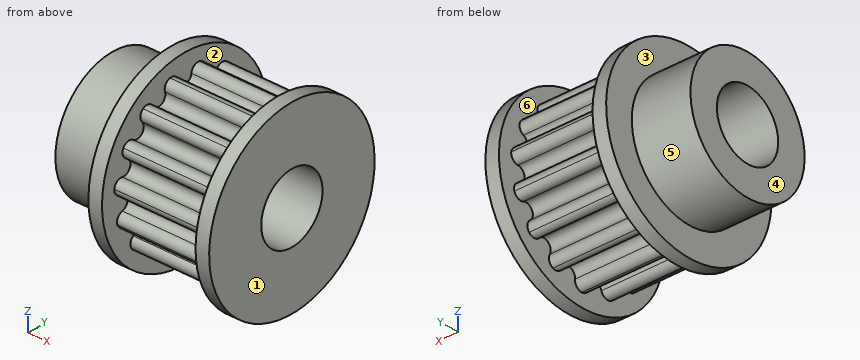
```python
from build123d import *

# Parameters (mm, degrees)
CUT_EXTRUDE1_START = 11
CUT_EXTRUDE1_DEPTH = 11


with BuildPart() as part:
    # Sketch1 → Revolve2 (revolve)
    with BuildSketch(Plane.XY, mode=Mode.PRIVATE) as revolve2_sk:
        Polygon((0, 4), (0, 7.45), (6.9, 7.45), (6.9, 10.8), (8.5, 10.8), (8.5, 9.25), (19.5, 9.25), (19.5, 10.8), (21.1, 10.8), (21.1, 4), align=None)
    revolve(revolve2_sk.sketch.rotate(Axis((0, 0, 0), (1, 0, 0)), 90), axis=Axis((0, 0, 0), (1, 0, 0)))

    # Sketch4 → Cut-Extrude1 (cut)
    with BuildSketch(Plane(origin=(8.5, 0, 0), x_dir=(0, 0, -1), z_dir=(1, 0, 0)).offset(CUT_EXTRUDE1_START)):
        with BuildLine():
            ThreePointArc((7.212898178, 4.164368705), (7.921100382, 4.238803586), (8.450295822, 3.762313188))
            ThreePointArc((8.450295822, 3.762313188), (7.483407656, 5.437012953), (6.189458648, 6.87408915))
            ThreePointArc((6.189458648, 6.87408915), (6.479096404, 6.223551012), (6.189458109, 5.573013113))
            ThreePointArc((6.189458109, 5.573013113), (6.067003582, 4.40793612), (7.212898178, 4.164368705))
        make_face()
        with BuildLine():
            ThreePointArc((8.283111715, 0.870590122), (8.960361705, 0.650538261), (9.25, 0))
            ThreePointArc((9.25, 0), (9.047865393, 1.923182733), (8.450295822, 3.762313188))
            ThreePointArc((8.450295822, 3.762313188), (8.450295314, 3.050210787), (7.921099986, 2.573721401))
            ThreePointArc((7.921099986, 2.573721401), (7.335352705, 1.55917735), (8.283111715, 0.870590122))
        make_face()
        with BuildLine():
            ThreePointArc((8.450295822, -3.762313187), (9.047865393, -1.923182732), (9.25, 0))
            ThreePointArc((9.25, 0), (8.960361705, -0.650538261), (8.283111715, -0.870590122))
            ThreePointArc((8.283111715, -0.870590122), (7.335352705, -1.55917735), (7.921099986, -2.573721401))
            ThreePointArc((7.921099986, -2.573721401), (8.450295314, -3.050210786), (8.450295822, -3.762313187))
        make_face()
        with BuildLine():
            ThreePointArc((6.189458648, -6.87408915), (7.483407656, -5.437012953), (8.450295822, -3.762313187))
            ThreePointArc((8.450295822, -3.762313187), (7.921100382, -4.238803585), (7.212898178, -4.164368705))
            ThreePointArc((7.212898178, -4.164368705), (6.067003582, -4.40793612), (6.189458109, -5.573013113))
            ThreePointArc((6.189458109, -5.573013113), (6.479096404, -6.223551011), (6.189458648, -6.87408915))
        make_face()
        with BuildLine():
            ThreePointArc((2.858407704, -8.797272611), (4.625000545, -8.010734671), (6.189458648, -6.87408915))
            ThreePointArc((6.189458648, -6.87408915), (5.512208479, -7.094141535), (4.89550902, -6.738090106))
            ThreePointArc((4.89550902, -6.738090106), (3.749614424, -6.494522691), (3.387602695, -7.608680229))
            ThreePointArc((3.387602695, -7.608680229), (3.387602803, -8.320782767), (2.858407704, -8.797272611))
        make_face()
        with BuildLine():
            ThreePointArc((-0.966888273, -9.199327533), (0.966888556, -9.199327504), (2.858407704, -8.797272611))
            ThreePointArc((2.858407704, -8.797272611), (2.15020562, -8.722837899), (1.731641877, -8.146734514))
            ThreePointArc((1.731641877, -8.146734514), (0.783882867, -7.458147287), (0, -8.32873741))
            ThreePointArc((0, -8.32873741), (-0.28963829, -8.979275667), (-0.966888273, -9.199327533))
        make_face()
        with BuildLine():
            ThreePointArc((-4.625000007, -8.010734981), (-2.858407196, -8.797272776), (-0.966888273, -9.199327533))
            ThreePointArc((-0.966888273, -9.199327533), (-1.58358738, -8.843276147), (-1.731641877, -8.146734514))
            ThreePointArc((-1.731641877, -8.146734514), (-2.317389159, -7.132190463), (-3.387602695, -7.608680229))
            ThreePointArc((-3.387602695, -7.608680229), (-3.916798196, -8.085169996), (-4.625000007, -8.010734981))
        make_face()
        with BuildLine():
            ThreePointArc((-7.483407198, -5.437013584), (-6.189458111, -6.874089633), (-4.625000007, -8.010734981))
            ThreePointArc((-4.625000007, -8.010734981), (-5.043563514, -7.434631729), (-4.89550902, -6.738090106))
            ThreePointArc((-4.89550902, -6.738090106), (-5.017963546, -5.573013113), (-6.189458109, -5.573013113))
            ThreePointArc((-6.189458109, -5.573013113), (-6.866708099, -5.793064974), (-7.483407198, -5.437013584))
        make_face()
        with BuildLine():
            ThreePointArc((-9.047865313, -1.923183112), (-8.450295489, -3.762313935), (-7.483407198, -5.437013584))
            ThreePointArc((-7.483407198, -5.437013584), (-7.631461691, -4.740471957), (-7.212898178, -4.164368705))
            ThreePointArc((-7.212898178, -4.164368705), (-6.85088645, -3.050211167), (-7.921099986, -2.573721401))
            ThreePointArc((-7.921099986, -2.573721401), (-8.629301806, -2.499286385), (-9.047865313, -1.923183112))
        make_face()
        with BuildLine():
            ThreePointArc((-8.283111715, 0.870590122), (-8.899810818, 1.226641519), (-9.047865304, 1.923183154))
            ThreePointArc((-9.047865304, 1.923183154), (-9.25, 2.2e-08), (-9.047865313, -1.923183112))
            ThreePointArc((-9.047865313, -1.923183112), (-8.899810805, -1.226641501), (-8.283111715, -0.870590122))
            ThreePointArc((-8.283111715, -0.870590122), (-7.499228848, 0), (-8.283111715, 0.870590122))
        make_face()
        with BuildLine():
            ThreePointArc((-7.212898178, 4.164368705), (-7.631461691, 4.740471957), (-7.483407198, 5.437013584))
            ThreePointArc((-7.483407198, 5.437013584), (-8.45029548, 3.762313955), (-9.047865304, 1.923183154))
            ThreePointArc((-9.047865304, 1.923183154), (-8.629301788, 2.499286395), (-7.921099986, 2.573721401))
            ThreePointArc((-7.921099986, 2.573721401), (-6.85088645, 3.050211167), (-7.212898178, 4.164368705))
        make_face()
        with BuildLine():
            ThreePointArc((-4.89550902, 6.738090106), (-5.043563514, 7.434631729), (-4.625000007, 8.010734981))
            ThreePointArc((-4.625000007, 8.010734981), (-6.189458111, 6.874089633), (-7.483407198, 5.437013584))
            ThreePointArc((-7.483407198, 5.437013584), (-6.866708099, 5.793064974), (-6.189458109, 5.573013113))
            ThreePointArc((-6.189458109, 5.573013113), (-5.017963546, 5.573013113), (-4.89550902, 6.738090106))
        make_face()
        with BuildLine():
            ThreePointArc((-1.731641877, 8.146734514), (-1.583587386, 8.843276139), (-0.966888291, 9.199327532))
            ThreePointArc((-0.966888291, 9.199327532), (-2.858407204, 8.797272774), (-4.625000007, 8.010734981))
            ThreePointArc((-4.625000007, 8.010734981), (-3.916798196, 8.085169996), (-3.387602695, 7.608680229))
            ThreePointArc((-3.387602695, 7.608680229), (-2.317389159, 7.132190463), (-1.731641877, 8.146734514))
        make_face()
        with BuildLine():
            ThreePointArc((1.731641877, 8.146734514), (2.15020538, 8.72283776), (2.858407176, 8.797272783))
            ThreePointArc((2.858407176, 8.797272783), (0.966888271, 9.199327534), (-0.966888291, 9.199327532))
            ThreePointArc((-0.966888291, 9.199327532), (-0.289638297, 8.979275673), (0, 8.32873741))
            ThreePointArc((0, 8.32873741), (0.783882867, 7.458147287), (1.731641877, 8.146734514))
        make_face()
        with BuildLine():
            ThreePointArc((4.89550902, 6.738090106), (5.512208479, 7.094141535), (6.189458648, 6.87408915))
            ThreePointArc((6.189458648, 6.87408915), (4.625000304, 8.010734809), (2.858407176, 8.797272783))
            ThreePointArc((2.858407176, 8.797272783), (3.38760269, 8.320783021), (3.387602695, 7.608680229))
            ThreePointArc((3.387602695, 7.608680229), (3.749614424, 6.494522691), (4.89550902, 6.738090106))
        make_face()
    extrude(amount=-CUT_EXTRUDE1_DEPTH, mode=Mode.SUBTRACT)


solid = part.part
```
Here's how the part is built. I have some questions about the finished solid (model axes, mm). Face numbers are marked on the shaded views. A direction names the side the tool comes from. Round coordinates to 2 decimals unless told otherwise and drop trailing zeros. Write each loop counter-clockwise with the first axis right and the second up, starting at its lowest first coordinate (ties: lowest second). Pieces come first, ordered by that corner, then holes.
Q1. If we section it at A-A on z = 2.5: Write out the boundary of the cut face in (x, y).
Q2. Which directions (+Z, -Z, +X, -X, +Y, -Y) give clear straight access to the entire face, cutting with the end or side of a thin tool? Please do the marked faces 1, 2 and 3.
Q3. If we section it at B-B on x = 1.5: Write out the boundary of the cut face in (y, z), plus the area to 3 significant figures.
Q4. If we mould it in two halves opening along X, with no side actions, what happens to the marked faces 4, 5 and 6? For each: +X half, -X half, draft (parallel to the pull), parting line (faces both ways), or undercut.
Q5. Please list where these lines run through material, in increasing order: probe 1 along X at (y, z) = (-1, -8.5); probe 2 along Y at (x, z) = (8, 0); probe 3 along Y at (x, z) = (18.75, -5.75).
Q6. Will these pins go through, and if not, where does the flat tip stop? P1, Ø2, axis at x = 18, z = 5.5, coming from the +Y side; P2, Ø10, axis at x = 11, z = -6, coming from the +Y side; P3, Ø2, axis at y = 4, z = -8.5, coming from the -X side; P4, Ø7, axis at y = 0, z = 0, coming from the -X side.
Answer below:
1. outline: (0, -7.02) - (6.9, -7.02) - (6.9, -10.51) - (8.5, -10.51) - (8.5, -7.09) - (19.5, -7.09) - (19.5, -10.51) - (21.1, -10.51) - (21.1, -3.12) - (0, -3.12) - close; (0, 3.12) - (21.1, 3.12) - (21.1, 10.51) - (19.5, 10.51) - (19.5, 7.09) - (8.5, 7.09) - (8.5, 10.51) - (6.9, 10.51) - (6.9, 7.02) - (0, 7.02) - close
2. face 1: +Z, -Z, +X, +Y, -Y
2. face 2: none
2. face 3: -X
3. outline: circle Ø14.9 at (0, 0); hole circle Ø8 at (0, 0)
3. area: 124 mm2
4. face 4: -X half
4. face 5: draft
4. face 6: undercut
5. probe 1: x = 6.9 to 8.5, 19.5 to 21.1
5. probe 2: y = -10.8 to -4, 4 to 10.8
5. probe 3: y = -7.09 to 7.09
6. P1: stops at y = 8.07
6. P2: stops at y = 10.67
6. P3: stops at x = 6.9
6. P4: passes through
